Autodesk Inventor part; units mm, degrees
ref_plane "YZ Plane" through (0, 0, 0) normal (1, 0, 0) x (0, 1, 0)
ref_plane "XZ Plane" through (0, 0, 0) normal (0, 1, 0) x (-1, 0, 0)
ref_plane "XY Plane" through (0, 0, 0) normal (0, 0, 1) x (1, 0, 0)
sketch "Sketch1" plane through (0, 0, 0) normal (0, 1, 0) x (-1, 0, 0)
  line L0 (0, 0) -> (254, 0)
  line L1 (254, 0) -> (254, 152.4)
  line L2 (254, 152.4) -> (0, 152.4)
  line L3 (0, 152.4) -> (0, 0)
  dimension "d0" = 254
  dimension "d1" = 152.4
extrude "Extrusion1" add sketch "Sketch1" against normal blind 12.7
sketch "Sketch5" plane through (0, -12.7, 0) normal (0, -1, 0) x (1, 0, 0)
  line L0 (0, 0) -> (0, 152.4)
  line L1 (0, 152.4) -> (-254, 152.4)
  line L2 (-254, 152.4) -> (-254, 0)
  point P0 (-38.1, 101.6)
  point P1 (-215.9, 101.6)
  dimension "d20" = 50.8
  dimension "d21" = 38.1
  dimension "d22" = 38.1
hole "Hole1" at (-38.1, -12.7, 101.6) at (-215.9, -12.7, 101.6) direction (0, 1, 0) diameter 6.35 end through all
sketch "Sketch10" plane through (0, 0, 0) normal (0, 1, 0) x (1, 0, 0)
  line L0 (-254, 0) -> (-254, -152.4)
  line L1 (-254, -152.4) -> (0, -152.4)
  line L2 (0, -152.4) -> (0, 0)
  point P0 (-88.9, -107.95)
  point P1 (-127, -107.95)
  point P2 (-165.1, -107.95)
  point P3 (-146.05, -133.35)
  point P4 (-107.95, -133.35)
  dimension "d67" = 38.1
  dimension "d69" = 38.1
  dimension "d70" = 19.05
  dimension "d71" = 19.05
  dimension "d72" = 127
  dimension "d73" = 127
  dimension "d74" = 19.05
  dimension "d75" = 25.4
hole "Hole5" at (-88.9, 0, 107.95) at (-127, 0, 107.95) at (-165.1, 0, 107.95) at (-146.05, 0, 133.35) at (-107.95, 0, 133.35) direction (0, -1, 0) diameter 6.35 end through all
properties part number "tractor"
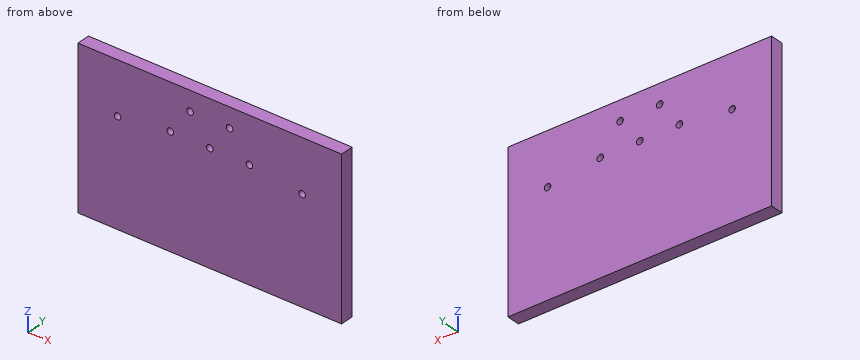
Model file for the job. Use its own axes, mm. Give positions to 0.01 mm unless a question says otherwise; leave off trailing zeros. Write each loop counter-clockwise with the first axis right and the second up, starting at its lowest first coordinate (ties: lowest second). Pieces come first, ordered by that corner, then holes. Notation, with made-up numbers: M 32.5,-39 L 88.5,-39 A17 cw 88.5,-26 Z; hole C 19,-4.5 d7. An arc over 180 degrees is marked long. One line per item, written item: value. Start each with the question number.
Q1. Probe probe 1 along X at (y, z) = (-4.75, 101.6) (3 decimals); probe 2 along X at (y, z) = (-6, 107.95) (3 decimals); probe 3 along Z at (x, y) = (-215.9, -10) (3 decimals). List the from-to ranges inside material, lowest first. Write a range as [from, to].
Q2. Saw through at C-C, the plane x = -107.95. Write the cut outline in (y, z) (3 decimals), plus the area to 3 significant figures.
Q3. Saw through at B-B, the plane z = 107.95. Write the cut outline in (x, y) (3 decimals).
Q4. Saw through at A-A, the plane z = 133.35. Write the cut outline in (x, y) (3 decimals).
Output values:
1. probe 1: x = [-254, -219.075], [-212.725, -41.275], [-34.925, 0]
1. probe 2: x = [-254, -168.275], [-161.925, -130.175], [-123.825, -92.075], [-85.725, 0]
1. probe 3: z = [0, 98.425], [104.775, 152.4]
2. outline: M -12.7,0 L 0,0 L 0,130.175 L -12.7,130.175 Z; M -12.7,136.525 L 0,136.525 L 0,152.4 L -12.7,152.4 Z
2. area: 1,850 mm²
3. outline: M -254,-12.7 L -168.275,-12.7 L -168.275,0 L -254,0 Z; M -161.925,-12.7 L -130.175,-12.7 L -130.175,0 L -161.925,0 Z; M -123.825,-12.7 L -92.075,-12.7 L -92.075,0 L -123.825,0 Z; M -85.725,-12.7 L 0,-12.7 L 0,0 L -85.725,0 Z
4. outline: M -254,-12.7 L -149.225,-12.7 L -149.225,0 L -254,0 Z; M -142.875,-12.7 L -111.125,-12.7 L -111.125,0 L -142.875,0 Z; M -104.775,-12.7 L 0,-12.7 L 0,0 L -104.775,0 Z
